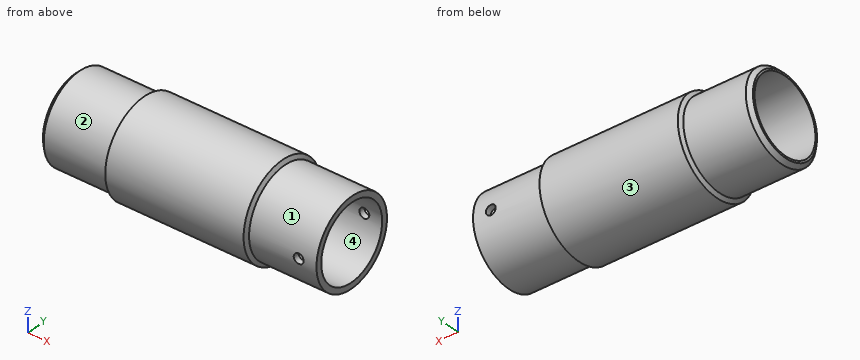
Autodesk Inventor part; units mm, degrees
ref_plane "YZ Plane" through (0, 0, 0) normal (1, 0, 0) x (0, 1, 0)
ref_plane "XZ Plane" through (0, 0, 0) normal (0, 1, 0) x (-1, 0, 0)
ref_plane "XY Plane" through (0, 0, 0) normal (0, 0, 1) x (1, 0, 0)
sketch "Profile" plane through (0, 0, 0) normal (0, 0, 1) x (1, 0, 0)
  line L0 (-16.8, 0) -> (-16.8, 11)
  line L1 (-16.8, 11) -> (0, 11)
  line L2 (0, 11) -> (0.5774, 12)
  line L3 (0.5774, 12) -> (35.5774, 12)
  line L4 (35.5774, 12) -> (36.1547, 11)
  line L5 (36.1547, 11) -> (53.2, 11)
  line L6 (53.2, 11) -> (53.2, 0)
  line L7 (-16.8, 0) -> (0, 0)
  line L8 (0, 0) -> (0, 9)
  line L9 (0, 9) -> (45.2, 9)
  line L10 (45.2, 9) -> (45.2, 0)
  line L11 (45.2, 0) -> (53.2, 0)
  line L12 (-30.8, 0) -> (67.2, 0) construction
  line L13 (0, 11) -> (0, 9) construction
  dimension "BodyLength" = 70
  dimension "d1" = 11
  dimension "d3" = 120
  dimension "d4" = 120
  dimension "d5" = 35
  dimension "d6" = 16.8
  dimension "d16" = 8
  dimension "d29" = 1
  dimension "d30" = 9
revolve "ProfileRevolveFeature" add sketch "Profile" angle 360 about axis through (-10, 0, 0) along (1, 0, 0)
sketch "InsideHole" plane through (-16.8, 0, 0) normal (-1, 0, 0) x (0, 0, 1)
  circle A0 centre (0, 0) radius 9 construction
hole "InsideHoleFeature" at (-16.8, 0, 0) direction (1, 0, 0) diameter 19 end through all
chamfer "EndChamferFeature" distance 1 angle 45 1 edges at (-16.8, -11, 0)
sketch "CapMountHole" plane through (0, 0, 0) normal (0, 1, 0) x (-1, 0, 0)
  line L0 (-53.2, 11) -> (-53.2, -11) construction
  line L1 (11.4, 0) -> (-68.4, 0) construction
  circle A0 centre (-48.7, 0) radius 1.25
  point P0 (0, 0)
  dimension "d31" = 4.5
  dimension "d39" = 2.5
extrude "CapMountHoleFeature" cut sketch "CapMountHole" along normal through all both and the other way through all
equation "\"d5\" = 0.5 * BodyLength"
equation "\"d6\" = 0.24 * BodyLength"
properties part number "BackPair1PistonBody"
CAD build for the part. Positions are in the model's coordinates, mm. Face numbers are marked on the shaded views. A direction names the side the tool comes from. Round coordinates to 2 decimals unless told otherwise and drop trailing zeros. Order: outer loops, then holes, each group sorted by start corner. A loop starts at its lowest first (then second) coordinate and runs counter-clockwise, first axis right, second up.
Q1. Slice it at C-C (x = 48.7). Write the cut outline in (y, z).
Q2. Which spindle directions (+Z, -Z, +X, -X, +Y, -Y) get a long thin tool onto all of the face, cutting with end or side? Do the marked faces 1 and 2. Say none if no direction does.
Q3. Drop flat-ended pins along their axis: pin 1 (4 mm diameter, centred on x = 48.7, z = 0, fed in from -Y); pin 2 (4 mm diameter, centred on x = -9, z = 4.5, fed in from +Y); pin 3 (8 mm diameter, centred on y = 6.5, z = 0.5, fed in from -X); pin 4 (1 mm diameter, centred on x = 35.5, y = 1.5, fed in from -Z). Give the stop position or say it passes through.
Q4. Slice it at D-D (x = 5.5). Write the cut outline in (y, z).
Q5. Wall check: L1, parallel to Z at x = 35.5, y = 0; L2, parallel to Y at x = 12.5, z = -2.5; L3, parallel to Y at x = 5.5, z = -5.75. Give the ranges that are in metal, low to high.
Q6. Two-plate mould, pull along Y, no slides. Class the marked faces 3 and 4: pulls with the +Y half, pulls with the -Y half, needs draft (parallel to the pull), parting line crosses it, or undercut.
Q7. Slice it at B-B (y = 0). Write the cut outline in (x, z).
Q8. Slice it at A-A (z = 0). Write the cut outline in (x, y).
Results below:
1. outline: (-10.93, -1.25) arc R11 ccw to (10.93, -1.25) - (9.42, -1.25) arc R9.5 cw to (-9.42, -1.25) - close; (-10.93, 1.25) - (-9.42, 1.25) arc R9.5 cw to (9.42, 1.25) - (10.93, 1.25) arc R11 ccw to start
2. face 1: +X
2. face 2: -X
3. pin 1: stops at y = -11
3. pin 2: stops at y = 10.71
3. pin 3: stops at x = -16.8
3. pin 4: stops at z = -11.96
4. outline: circle Ø24 at (0, 0); hole circle Ø19 at (0, 0)
5. L1: z = -12 to -9.5, 9.5 to 12
5. L2: y = -11.74 to -9.17, 9.17 to 11.74
5. L3: y = -10.53 to -7.56, 7.56 to 10.53
6. face 3: parting line crosses it
6. face 4: undercut
7. outline: (-16.8, -10) - (-15.8, -11) - (0, -11) - (0.58, -12) - (35.58, -12) - (36.15, -11) - (53.2, -11) - (53.2, -9.5) - (-16.8, -9.5) - close; (-16.8, 9.5) - (53.2, 9.5) - (53.2, 11) - (36.15, 11) - (35.58, 12) - (0.58, 12) - (0, 11) - (-15.8, 11) - (-16.8, 10) - close
8. outline: (-16.8, -10) - (-15.8, -11) - (0, -11) - (0.58, -12) - (35.58, -12) - (36.15, -11) - (47.45, -11) - (47.45, -9.5) - (-16.8, -9.5) - close; (-16.8, 9.5) - (47.45, 9.5) - (47.45, 11) - (36.15, 11) - (35.58, 12) - (0.58, 12) - (0, 11) - (-15.8, 11) - (-16.8, 10) - close; (49.95, -11) - (53.2, -11) - (53.2, -9.5) - (49.95, -9.5) - close; (49.95, 9.5) - (53.2, 9.5) - (53.2, 11) - (49.95, 11) - close
